Autodesk Inventor part; units mm, degrees
ref_plane "YZ Plane" through (0, 0, 0) normal (1, 0, 0) x (0, 1, 0)
ref_plane "XZ Plane" through (0, 0, 0) normal (0, 1, 0) x (-1, 0, 0)
ref_plane "XY Plane" through (0, 0, 0) normal (0, 0, 1) x (1, 0, 0)
sketch "Sketch1" plane through (0, 0, 0) normal (0, 0, 1) x (1, 0, 0)
  line L0 (-100, 100) -> (100, 100)
  line L1 (100, 100) -> (100, -100)
  line L2 (100, -100) -> (-100, -100)
  line L3 (-100, -100) -> (-100, 100)
  line L4 (-100, 100) -> (100, -100) construction
  line L5 (100, 100) -> (-100, -100) construction
  point P0 (0, 0)
  point P1 (0, 0)
  point P2 (0, 0)
  dimension "d25" = 200
  dimension "d26" = 200
extrude "Plate1" add sketch "Sketch1" along normal blind 3
sketch "Sketch6" plane through (0, 0, 3) normal (0, 0, 1) x (1, 0, 0)
  circle A0 centre (-75, 0) radius 15
  circle A1 centre (75, 0) radius 15
  line L0 (0, 0) -> (0, 55.0725) construction
  dimension "d37" = 30
  dimension "d38" = 150
cut "Cut1" [suppressed]
sketch "Sketch8" plane through (0, 0, 0) normal (1, 0, 0) x (0, 1, 0)
  line L0 (-94.2929, 40) -> (94.2929, 40)
  circle A0 centre (0, 30) radius 6.5
  line L1 (89.2929, 5) -> (-89.2929, 5)
  point P0 (0, 0)
  dimension "d48" = 13
  dimension "d49" = 25
extrude "Extrusion3" [suppressed]
pattern_linear "Rectangular Pattern2" [suppressed]
sketch "Sketch9" plane through (0, 0, 3) normal (0, 0, 1) x (1, 0, 0)
  circle A0 centre (-65, 65) radius 6.5
  point P0 (0, 0)
  point P1 (-225, 65)
  dimension "d55" = 13
  dimension "d73" = 65
  dimension "d74" = 65
extrude "Cut2" cut sketch "Sketch9" against normal blind 3
mirror "Mirror1" about plane through (0, 0, 0) normal (1, 0, 0) of "Cut2"
mirror "Mirror2" about plane through (0, 0, 0) normal (0, 1, 0) of "Cut2", "Mirror1"
sketch "Sketch10" plane through (0, 0, 0) normal (0, 0, -1) x (-1, 0, 0)
  circle A0 centre (0, 0) radius 25
  dimension "d75" = 50
extrude "Cut3" cut sketch "Sketch10" against normal blind 3
equation "\"d26\" = Гриндер_высота"
equation "\"d38\" = Гриндер_Валы_между_центрами"
equation "\"d39\" = Thickness"
equation "\"d48\" = Гриндер_диам_отврс_корпуса"
equation "\"d49\" = Гриндер_отступ_отврс_корпуса"
equation "\"d55\" = Гриндер_диам_отврс_корпуса"
equation "\"d57\" = Thickness"
equation "\"d76\" = Thickness"
equation "\"d2\" = Thickness"
equation "\"BendReliefWidth\" = Thickness"
equation "\"BendReliefDepth\" = 0.5 * Thickness"
equation "\"CornerReliefSize\" = 4 * Thickness"
equation "\"MinimumRemnant\" = 2 * Thickness"
equation "\"TransitionRadius\" = BendRadius"
equation "\"JacobiRadiusSize\" = BendRadius"
equation "\"GapSize\" = Thickness"
equation "\"Гриндер_отступ_отврс_корпуса\" = 25"
equation "\"Гриндер_диам_отврс_корпуса\" = 13"
equation "\"Гриндер_высота\" = 200"
equation "\"Гриндер_Валы_между_центрами\" = 150"
properties part number "NDM-VOS 777 sredder wall 7" material "Stainless Steel"
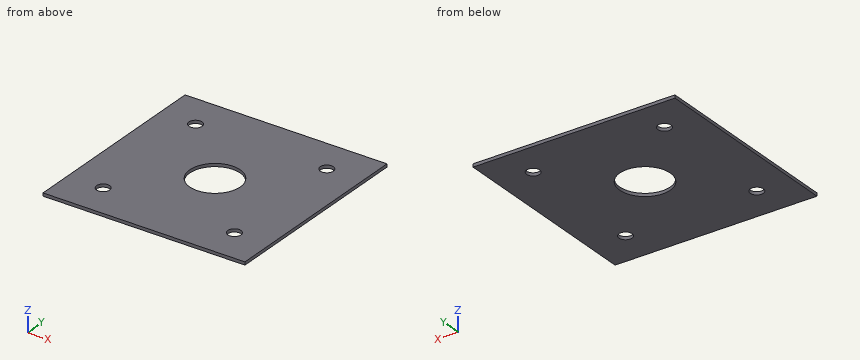
The model under review builds one solid part; all positions refer to its coordinate system, in mm. Round coordinates to 2 decimals unless told otherwise and drop trailing zeros. Loops run counter-clockwise (first coordinate to the right, second up) from the corner with the lowest first, then second, coordinate; pieces in that order, holes last. Notation, with made-up numbers: M 21,53 L 54,53 A23 cw 54,76 Z; hole C 6.5,49.5 d1. An arc over 180 degrees is marked long. Answer as a JSON object with one key per item and string values.
(1) Take a section at A-A on x = 0. Give the boundary of the cut face in (y, z), and give its area (3 significant figures).
Resolved:
{"outline": "M -100,0 L -25,0 L -25,3 L -100,3 Z; M 25,0 L 100,0 L 100,3 L 25,3 Z", "area": "450 mm²"}
(2) Take a section at C-C on z = 2.55. Give the boundary of the cut face in (x, y), and give its area (3 significant figures).
Resolved:
{"outline": "M -100,-100 L 100,-100 L 100,100 L -100,100 Z; hole C -65,-65 d13; hole C -65,65 d13; hole C 0,0 d50; hole C 65,-65 d13; hole C 65,65 d13", "area": "37,500 mm²"}
(3) Clearance check with a flat-ended pin moving along its axis: P1, Ø8, axis at x = -65, y = -65, coming from the +Z side. State where the tip first meets the part, or that it passes through.
Resolved:
{"P1": "through"}
(4) Take a section at B-B on y = 65. Give the boundary of the cut face in (x, z).
Resolved:
{"outline": "M -100,0 L -71.5,0 L -71.5,3 L -100,3 Z; M -58.5,0 L 58.5,0 L 58.5,3 L -58.5,3 Z; M 71.5,0 L 100,0 L 100,3 L 71.5,3 Z"}
(5) To check wall thickness, follow line 1 along Y through (x, z) = (-65, 1.05); line 2 along Y through (x, z) = (0, 0.7). State the ranges of each line that lie inside material, in increasing order.
Resolved:
{"line 1": "-100 to -71.5, -58.5 to 58.5, 71.5 to 100", "line 2": "-100 to -25, 25 to 100"}
